Design review of the part built by this model. Coordinates are the model's own, in mm. Round coordinates to 2 decimals unless told otherwise and drop trailing zeros. Write each loop counter-clockwise with the first axis right and the second up, starting at its lowest first coordinate (ties: lowest second). Pieces come first, ordered by that corner, then holes.
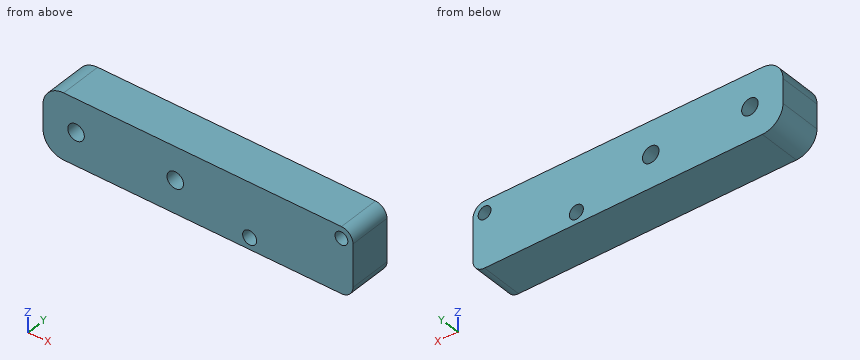
from build123d import *

# Parameters (mm, degrees)
F0_W     = 27.8
F0_H     = 15.9
F1_DEPTH = 10.3
F2_R     = 1.7
F2_R_2   = 1.55
F3_DEPTH = 10.301
F4_R     = 2.8
F6_DEPTH = 10.3
F7_R     = 2
F8_DEPTH = 10.3


with BuildPart() as f1:
    # F0 (on Front) → F1 (new body)
    with BuildSketch(Plane.XZ):
        with Locations((13.9, 7.95)):
            Rectangle(F0_W, F0_H)
    extrude(amount=F1_DEPTH)

    # F2 (on face) → F3 (cut, through all)
    with BuildSketch(Plane.XZ.offset(10.3)):
        with Locations((2.8, 2.8)):
            Circle(F2_R)
        with Locations((25, 13.1)):
            Circle(F2_R_2)
    extrude(amount=-F3_DEPTH, mode=Mode.SUBTRACT)

    # F4
    f4_edges = [f1.edges().sort_by_distance(p)[0] for p in [
        (0, -5.15, 0),
        (0, -5.15, 15.9),
        (27.8, -5.15, 0),
        (27.8, -5.15, 15.9),
    ]]
    fillet(f4_edges, radius=F4_R)

    # F5 (on face) → F6 (join, through all)
    with BuildSketch(Plane.XZ.offset(10.3)):
        with BuildLine():
            ThreePointArc((0, 13.1), (0.820101, 15.079899), (2.8, 15.9))
            Line((2.8, 15.9), (-42.2, 15.9))
            ThreePointArc((-42.2, 15.9), (-45.735534, 14.435534), (-47.2, 10.9))
            Line((-47.2, 10.9), (-47.2, 5))
            ThreePointArc((-47.2, 5), (-45.735534, 1.464466), (-42.2, 0))
            Line((-42.2, 0), (2.8, 0))
            ThreePointArc((2.8, 0), (0.820101, 0.820101), (0, 2.8))
            Line((0, 2.8), (0, 13.1))
        make_face()
    extrude(amount=-F6_DEPTH)

    # F7 (on face) → F8 (cut, through all)
    with BuildSketch(Plane(origin=(0, 0, 0), x_dir=(-1, 0, 0), z_dir=(0, 1, 0))):
        with Locations((39.2, 7.95)):
            Circle(F7_R)
        with Locations((15.2, 7.95)):
            Circle(F7_R)
    extrude(amount=-F8_DEPTH, mode=Mode.SUBTRACT)


solid = f1.part
1) Add section C-C on x = 2.8. State the section outline as (y, z) points, and give its area (3 significant figures).
2) Add section B-B on z = 7.95. State the section outline as (x, y) points.
3) Add section D-D on z = 13.75. State the section outline as (x, y) points, and give its area (3 significant figures).
4) For line 1 along X through (y, z) = (-6, 7.75); line 2 along Z through (x, y) = (25, -2); line 3 along Z through (x, y) = (-39.2, -6.75), list the stretches that pass through material, from the lowest coordinate up.
5) Add section A-A on y = -0.75. State the section outline as (x, z) points, and give its area (3 significant figures).
Computed:
1. outline: (-10.3, 0) - (0, 0) - (0, 1.1) - (-10.3, 1.1) - close; (-10.3, 4.5) - (0, 4.5) - (0, 15.9) - (-10.3, 15.9) - close
1. area: 129 mm2
2. outline: (-47.2, -10.3) - (-41.2, -10.3) - (-41.2, 0) - (-47.2, 0) - close; (-37.2, -10.3) - (-17.2, -10.3) - (-17.2, 0) - (-37.2, 0) - close; (-13.2, -10.3) - (27.8, -10.3) - (27.8, 0) - (-13.2, 0) - close
3. outline: (-46.31, -10.3) - (23.59, -10.3) - (23.59, 0) - (-46.31, 0) - close; (26.41, -10.3) - (27.72, -10.3) - (27.72, 0) - (26.41, 0) - close
3. area: 734 mm2
4. line 1: x = -47.2 to -41.19, -37.21 to -17.19, -13.21 to 27.8
4. line 2: z = 0 to 11.55, 14.65 to 15.9
4. line 3: z = 0 to 5.95, 9.95 to 15.9
5. outline: (-47.2, 5) arc R5 ccw to (-42.2, 0) - (25, 0) arc R2.8 ccw to (27.8, 2.8) - (27.8, 13.1) arc R2.8 ccw to (25, 15.9) - (-42.2, 15.9) arc R5 ccw to (-47.2, 10.9) - close; hole circle Ø4 at (-39.2, 7.95); hole circle Ø4 at (-15.2, 7.95); hole circle Ø3.4 at (2.8, 2.8); hole circle Ø3.1 at (25, 13.1)
5. area: 1,140 mm2
